from build123d import *

# Parameters (mm, degrees)
SKETCH_1_W                 = 300
SKETCH_1_H                 = 30
EXTRUDE_1_DEPTH            = 5
CHAMFER_1_SIZE             = 1
HOLE_WIZARD_M3_1_D         = 3.2
M3X0_5_1_D                 = 2.5
M4X0_7_1_D                 = 3.3
M4X0_7_2_D                 = 3.3
PATTERN_LINEAR_1_COUNT     = 6
PATTERN_LINEAR_1_PITCH     = 25
PATTERN_LINEAR_1_COL_COUNT = 7
PATTERN_LINEAR_1_COL_PITCH = 25
EXTRUDE_3_DEPTH            = 5
SKETCH_13_R                = 3.6
CUT_EXTRUDE_2_DEPTH        = 161.542829177
HOLE_WIZARD_M2_5_1_D       = 2.7
M4X0_7_3_D                 = 3.3
HOLE_WIZARD_M4_1_D         = 4.3
M3X0_5_2_D                 = 2.5


with BuildPart() as part:
    # 草圖1 → 填料-伸長1 (new body)
    with BuildSketch(Plane.XY):
        Rectangle(SKETCH_1_W, SKETCH_1_H)
    extrude(amount=EXTRUDE_1_DEPTH)

    # 導角1
    chamfer_1_edges = [part.edges().sort_by_distance(p)[0] for p in [
        (150, -15, 2.5),
        (-150, -15, 2.5),
        (-150, 15, 2.5),
        (150, 15, 2.5),
    ]]
    chamfer(chamfer_1_edges, length=CHAMFER_1_SIZE)

    # M3 餘隙孔1 (through all)
    with Locations(Plane.XY.offset(5)):
        with Locations((20, -10), (20, 10), (0, -10), (0, 10)):
            Hole(HOLE_WIZARD_M3_1_D / 2)

    # M3x0.5 螺紋孔1 (through all)
    with Locations(Plane.XY.offset(5)):
        with Locations((-12.5, 0)):
            m3x0_5_1 = Hole(M3X0_5_1_D / 2)

    # M4x0.7 螺紋孔1 (through all)
    with Locations(Plane.XY.offset(5)):
        with Locations((80, 10), (50, -10), (50, 10), (80, -10), (65, 10), (65, -10)):
            Hole(M4X0_7_1_D / 2)

    # M4x0.7 螺紋孔2 (through all)
    with Locations(Plane.XY.offset(5)):
        with Locations((-126, 10), (-126, -10)):
            m4x0_7_2 = Hole(M4X0_7_2_D / 2)

    # 直線複製排列1: M3x0.5 螺紋孔1 ×6
    with Locations(*[(-i * PATTERN_LINEAR_1_PITCH, 0, 0) for i in range(1, PATTERN_LINEAR_1_COUNT)]):
        add(m3x0_5_1, mode=Mode.SUBTRACT)

    # 直線複製排列1 col: M3x0.5 螺紋孔1 ×7
    with Locations(*[(i * PATTERN_LINEAR_1_COL_PITCH, 0, 0) for i in range(1, PATTERN_LINEAR_1_COL_COUNT)]):
        add(m3x0_5_1, mode=Mode.SUBTRACT)

    # 鏡射1: M4x0.7 螺紋孔2 across plane
    add(m4x0_7_2.mirror(Plane(origin=(0, 0, 0), x_dir=(0, 0, 1), z_dir=(1, 0, 0))), mode=Mode.SUBTRACT)

    # 草圖16 → 填料-伸長3 (add, through all)
    with BuildSketch(Plane.XY):
        with BuildLine():
            Line((-20, 15), (44, 15))
            Line((44, 15), (44, 57))
            Line((44, 57), (0, 57))
            ThreePointArc((0, 57), (-14.142135624, 51.142135624), (-20, 37))
            Line((-20, 37), (-20, 15))
        make_face()
    extrude(amount=EXTRUDE_3_DEPTH)

    # 草圖13 → 除料-伸長2 (cut, through all)
    with BuildSketch(Plane.XY):
        with Locations(Location((34, 24.8, 0), (0, 0, 180))):
            Circle(SKETCH_13_R)
    extrude(amount=CUT_EXTRUDE_2_DEPTH, mode=Mode.SUBTRACT)

    # M2.5 餘隙孔1 (through all)
    with Locations(Plane.XY.offset(5)):
        with Locations((26.5, 24.8), (41.5, 24.8)):
            Hole(HOLE_WIZARD_M2_5_1_D / 2)

    # M4x0.7 螺紋孔3 (through all)
    with Locations(Plane.XY.offset(5)):
        with Locations((15, 22), (-15, 22)):
            Hole(M4X0_7_3_D / 2)

    # M4 餘隙孔1 (through all)
    with Locations(Plane.XY.offset(5)):
        with Locations((-26, -10), (-26, 10), (-50, -10), (-50, 10)):
            Hole(HOLE_WIZARD_M4_1_D / 2)

    # M3x0.5 螺紋孔2 (through all)
    with Locations(Plane.XY.offset(5)):
        with Locations((33, 53), (33, 45)):
            Hole(M3X0_5_2_D / 2)


solid = part.part
Model file for the job. Use its own axes, mm. A direction names the side the tool comes from. Coordinates: 2 decimals unless noted, no trailing zeros. Write each question's results on one line, items separated by ' | '. Start each with the question number.
1) Mould opens along Y. For faces 4 (the face through (-2, 14, 0)), 5 (the face through (-2, -15, 2)), 6 (the face through (34.78, 28.314, 2.465)), 7 (the face through (-13.986, 51.297, 2.465)) say: pulls with the +Y half, pulls with the -Y half, needs draft (parallel to the pull), parting line crosses it, or undercut.
2) Flat gauge pins, fed straight in: P1, Ø3, axis at x = 65, y = -10, coming from the +Z side; P2, Ø2, axis at y = 31.5, z = 3, coming from the -X side. Where does each tip first touch, or does it go through?
3) Probe line 1 along Y through (x, z) = (50, 3.95); line 2 along Y through (x, z) = (-48.5, 4.05); line 3 along Y through (x, z) = (71, 3.1). List the from-to ranges inside material, lowest first. Write a range as from..to.
4) 3-axis set-ups, long thin cutter, end or side, ignore diameter. For faces 1 (the face through (150, 0, 2)), 2 (the face through (-85, 15, 2)), 3 (the face through (44, 36, 2)): which of +Z, -Z, +X, -X, +Y, -Y reach the whole face in a straight line?
5) Cut at A-A (z = 2.85). Count the separate pieces of the cut face and the enclosed holes in it, then the cut area to 3 significant figures.
Returned:
1) face 4: needs draft | face 5: pulls with the -Y half | face 6: undercut | face 7: pulls with the +Y half
2) P1: through | P2: x = -20
3) line 1: -15..-11.65, -8.35..8.35, 11.65..15 | line 2: -15..-11.54, -8.46..8.46, 11.54..15 | line 3: -15..15
4) face 1: +Z, -Z, +X, +Y, -Y | face 2: +Z, -Z, -X, +Y | face 3: +Z, -Z, +X, +Y
5) separate pieces: 1 | enclosed holes: 37 | area: 11,300 mm^2
